from build123d import *

# Parameters (mm, degrees)
ESQUISSE3_R             = 2.55
STRUCTURE_DEPTH         = 9
ESQUISSE4_R             = 10
ESQUISSE4_R_2           = 11.5
ESQUISSE4_R_3           = 2.05
ENL_V_MAT_EXTRU_1_DEPTH = 10


with BuildPart() as part:
    # Esquisse3 → structure (new body)
    with BuildSketch(Plane(origin=(0, 0, 0), x_dir=(1, 0, 0), z_dir=(0, 1, 0))):
        Polygon((125, 110), (-125, 110), (-170, 95), (-170, 0), (-170, -120), (-150, -140), (-120, -140), (120, -140), (150, -140), (170, -120), (170, 0), (170, 95), align=None)
        with Locations(Location((-140, 80, 0), (0, 0, 270))):
            Circle(ESQUISSE3_R, mode=Mode.SUBTRACT)
        with Locations(Location((-140, -80, 0), (0, 0, 90))):
            Circle(ESQUISSE3_R, mode=Mode.SUBTRACT)
        with Locations(Location((140, -80, 0), (0, 0, 270))):
            Circle(ESQUISSE3_R, mode=Mode.SUBTRACT)
        with Locations(Location((140, 80, 0), (0, 0, 90))):
            Circle(ESQUISSE3_R, mode=Mode.SUBTRACT)
    extrude(amount=-STRUCTURE_DEPTH)

    # Esquisse4 → Enlèv. mat.-Extru.1 (cut)
    with BuildSketch(Plane(origin=(0, 0, 0), x_dir=(1, 0, 0), z_dir=(0, 1, 0))):
        with Locations(Location((0, 0, 0), (0, 0, 270))):
            Circle(ESQUISSE4_R)
        with Locations(Location((0, -80, 0), (0, 0, 270))):
            Circle(ESQUISSE4_R_2)
        with Locations(Location((0, 40, 0), (0, 0, 270))):
            Circle(ESQUISSE4_R_3)
        with Locations(Location((40, 0, 0), (0, 0, 270))):
            Circle(ESQUISSE4_R_3)
        with Locations(Location((0, -40, 0), (0, 0, 270))):
            Circle(ESQUISSE4_R_3)
        with Locations(Location((-40, 0, 0), (0, 0, 270))):
            Circle(ESQUISSE4_R_3)
    extrude(amount=-ENL_V_MAT_EXTRU_1_DEPTH, mode=Mode.SUBTRACT)


solid = part.part
The model under review builds one solid part; all positions refer to its coordinate system, in mm. Round coordinates to 2 decimals unless told otherwise and drop trailing zeros. Answer as a JSON object with one key per item and string values.
Item 1: The part is to be moulded in two halves that separate along X. For faces 1 (the face through (-9.76, -4.44, -2.17)), 2 (the face through (2, -4, -110)), 3 (the face through (-170, -4, 11)), say which applies: +X half, -X half, draft (parallel to the pull), parting line (faces both ways), or undercut.
Check sheet entries:
{"face 1": "undercut", "face 2": "draft", "face 3": "-X half"}
Item 2: Clearance check with a flat-ended pin moving along its axis: P1, Ø3.5, axis at x = 0, z = 40, coming from the -Y side. State where the tip first meets the part, or that it passes through.
Check sheet entries:
{"P1": "through"}
Item 3: We need section A-A, the plane y = -7.25. State how many separate pieces and enclosed holes the cut face has, and give its area (3 significant figures).
Check sheet entries:
{"separate pieces": "1", "enclosed holes": "10", "area": "83,100 mm2"}
Item 4: For line 1 along X through (y, z) = (-4, 80); line 2 along X through (y, z) = (-5, -80); line 3 along X through (y, z) = (-2, 0), list the stretches that pass through material, from the lowest coordinate up.
Check sheet entries:
{"line 1": "-170 to -142.55, -137.45 to -11.5, 11.5 to 137.45, 142.55 to 170", "line 2": "-170 to -142.55, -137.45 to 137.45, 142.55 to 170", "line 3": "-170 to -42.05, -37.95 to -10, 10 to 37.95, 42.05 to 170"}
